from build123d import *

# Parameters (mm, degrees)
X_WING_DEPTH       = 12.7
SKETCH4_3_R        = 1.5
SKETCH4_3_R_2      = 3.175
HOLES_DEPTH        = 9.525
CHIP_DEPTH         = 6.35
EXTRUDE_9V_DEPTH   = 15.24
SKETCH6_3_R        = 1.27
AIR_HOLES_DEPTH    = 9.525
SKETCH7_W          = 7.542953633
SKETCH7_H          = 7.880697826
SKETCH7_H_2        = 6.417139658
SKETCH7_W_2        = 5.741651273
SKETCH7_H_3        = 8.218442018
AIR_SLOTS_DEPTH    = 1.27
CUT_EXTRUDE1_START = 4.572
SKETCH4_5_R        = 1.5
CUT_EXTRUDE1_DEPTH = 0.508


with BuildPart() as part:
    # Sketch2 → Body (revolve)
    with BuildSketch(Plane(origin=(0, 0, 0), x_dir=(0, 0, -1), z_dir=(1, 0, 0))):
        Polygon((4.4704, 13.9065), (0, 12.5857), (0, 0), (-5.08, 0), (-5.08, 49.53), (64.831152593, 49.53), (64.831152593, 39.37), (59.751152593, 39.37), (59.751152593, 44.45), (0, 44.45), (0, 16.4465), (4.4704, 16.4465), align=None)
    revolve(axis=Axis((0, 0, 0), (0, 0, 1)))

    # Sketch4 → X-Wing (cut)
    with BuildSketch(Plane.XY):
        with BuildLine():
            Line((-4.1656, -12.04250002), (-4.1656, -10.483480973))
            ThreePointArc((-4.1656, -10.483480973), (-6.016064494, -6.016064494), (-10.483480973, -4.1656))
            Line((-10.483480973, -4.1656), (-16.265, -4.1656))
            ThreePointArc((-16.265, -4.1656), (-20.4306, 0), (-16.265, 4.1656))
            Line((-16.265, 4.1656), (-12.04250002, 4.1656))
            Line((-12.04250002, 4.1656), (-10.483480973, 4.1656))
            ThreePointArc((-10.483480973, 4.1656), (-6.016064494, 6.016064494), (-4.1656, 10.483480973))
            Line((-4.1656, 10.483480973), (-4.1656, 12.04250002))
            Line((-4.1656, 12.04250002), (-4.1656, 16.265))
            ThreePointArc((-4.1656, 16.265), (0, 20.4306), (4.1656, 16.265))
            Line((4.1656, 16.265), (4.1656, 12.04250002))
            Line((4.1656, 12.04250002), (4.1656, 10.483480973))
            ThreePointArc((4.1656, 10.483480973), (6.016064494, 6.016064494), (10.483480973, 4.1656))
            Line((10.483480973, 4.1656), (12.04250002, 4.1656))
            Line((12.04250002, 4.1656), (16.265, 4.1656))
            ThreePointArc((16.265, 4.1656), (20.4306, 0), (16.265, -4.1656))
            Line((16.265, -4.1656), (12.04250002, -4.1656))
            Line((12.04250002, -4.1656), (10.483480973, -4.1656))
            ThreePointArc((10.483480973, -4.1656), (6.016064494, -6.016064494), (4.1656, -10.483480973))
            Line((4.1656, -10.483480973), (4.1656, -12.04250002))
            Line((4.1656, -12.04250002), (4.1656, -16.265))
            ThreePointArc((4.1656, -16.265), (0, -20.4306), (-4.1656, -16.265))
            Line((-4.1656, -16.265), (-4.1656, -12.04250002))
        make_face()
    extrude(amount=-X_WING_DEPTH, mode=Mode.SUBTRACT)

    # Sketch4<3> → Holes (cut)
    with BuildSketch(Plane.XY):
        with Locations(Location((0, -16.265, 0), (0, 0, 180))):
            Circle(SKETCH4_3_R)
        with Locations(Location((-16.265, 0, 0), (0, 0, 180))):
            Circle(SKETCH4_3_R)
        with Locations(Location((16.265, 0, 0), (0, 0, 180))):
            Circle(SKETCH4_3_R)
        with Locations(Location((0, 16.265, 0), (0, 0, 180))):
            Circle(SKETCH4_3_R)
        with BuildLine():
            ThreePointArc((-7.633217703, 13.021371376), (-7.633217703, 17.511499436), (-12.123345763, 17.511499436))
            Line((-12.123345763, 17.511499436), (-17.511499436, 12.123345763))
            ThreePointArc((-17.511499436, 12.123345763), (-17.511499436, 7.633217703), (-13.021371376, 7.633217703))
            Line((-13.021371376, 7.633217703), (-7.633217703, 13.021371376))
        make_face()
        with Locations((-8.261128525, 8.261128525)):
            Circle(SKETCH4_3_R_2)
        with Locations(Location((8.261128525, 8.261128525, 0), (0, 0, 125.826899667))):
            Circle(SKETCH4_3_R_2)
        with Locations(Location((8.261128525, -8.261128525, 0), (0, 0, 234.173100333))):
            Circle(SKETCH4_3_R_2)
        with Locations(Location((-8.261128525, -8.261128525, 0), (0, 0, 144.173100333))):
            Circle(SKETCH4_3_R_2)
    extrude(amount=HOLES_DEPTH, mode=Mode.SUBTRACT)

    # Sketch6 → Chip (add)
    with BuildSketch(Plane.XY.offset(5.08)):
        Polygon((11.350015507, 22.225), (-11.715690517, 22.225), (-12.954, 22.225), (-12.954, 16.6808452), (-12.7, 16.9348452), (-12.7, 20.32), (12.7, 20.32), (12.7, -20.32), (-12.7, -20.32), (-12.7, 7.954589078), (-12.954, 7.700589078), (-12.954, -22.225), (12.954, -22.225), (12.954, 22.225), align=None)
    extrude(amount=CHIP_DEPTH)

    # Sketch6<4> → Extrude 9V (add)
    with BuildSketch(Plane.XY.offset(5.08)):
        Polygon((-14.859, 14.7758452), (-12.954, 16.6808452), (-12.954, 22.225), (-11.715690517, 22.225), (-11.715690517, 23.479848526), (-14.859, 23.479848526), align=None)
        with BuildLine():
            ThreePointArc((-13.021371376, 7.633217703), (-13.865328691, 7.029154679), (-14.859, 6.729532555))
            Line((-14.859, 6.729532555), (-14.859, 0.522650935))
            ThreePointArc((-14.859, 0.522650935), (-14.765, 0), (-14.859, -0.522650935))
            Line((-14.859, -0.522650935), (-14.859, -24.638))
            Line((-14.859, -24.638), (14.859, -24.638))
            Line((14.859, -24.638), (14.859, -0.522650935))
            ThreePointArc((14.859, -0.522650935), (14.765, 0), (14.859, 0.522650935))
            Line((14.859, 0.522650935), (14.859, 29.972))
            Line((14.859, 29.972), (-14.859, 29.972))
            Line((-14.859, 29.972), (-14.859, 28.067))
            Line((-14.859, 28.067), (12.954, 28.067))
            Line((12.954, 28.067), (12.954, 23.734213344))
            Line((12.954, 23.734213344), (11.350015507, 23.734213344))
            Line((11.350015507, 23.734213344), (11.350015507, 22.225))
            Line((11.350015507, 22.225), (12.954, 22.225))
            Line((12.954, 22.225), (12.954, -22.733))
            Line((12.954, -22.733), (-12.954, -22.733))
            Line((-12.954, -22.733), (-12.954, 7.700589078))
            Line((-12.954, 7.700589078), (-13.021371376, 7.633217703))
        make_face()
    extrude(amount=EXTRUDE_9V_DEPTH)

    # Sketch6<3> → Air holes (cut)
    with BuildSketch(Plane.XY.offset(5.08)):
        with Locations((-23.749, -23.368)):
            Circle(SKETCH6_3_R)
        with Locations((23.114, -15.748)):
            Circle(SKETCH6_3_R)
        with Locations((-9.906, 36.322)):
            Circle(SKETCH6_3_R)
        with Locations((18.034, 36.322)):
            Circle(SKETCH6_3_R)
    extrude(amount=-AIR_HOLES_DEPTH, mode=Mode.SUBTRACT)

    # Sketch7 → Air Slots (cut)
    with BuildSketch(Plane.XY.offset(5.08)):
        with Locations((15.537525525, 8.731732869)):
            Rectangle(SKETCH7_W, SKETCH7_H)
        with Locations((15.537525525, -8.324348854)):
            Rectangle(SKETCH7_W, SKETCH7_H_2)
        with Locations((-14.859451804, -9.225000034)):
            Rectangle(SKETCH7_W_2, SKETCH7_H_3)
    extrude(amount=AIR_SLOTS_DEPTH, mode=Mode.SUBTRACT)

    # SurfaceCut1
    split(bisect_by=Plane.XY.offset(5.08), keep=Keep.BOTTOM)

    # Sketch4<5> → Cut-Extrude1 (cut)
    with BuildSketch(Plane.XY.offset(CUT_EXTRUDE1_START)):
        with BuildLine():
            ThreePointArc((5.098211557, -7.98439534), (6.016064494, -6.016064494), (7.98439534, -5.098211557))
            ThreePointArc((7.98439534, -5.098211557), (9.203861468, -4.686142824), (10.483480973, -4.5466))
            Line((10.483480973, -4.5466), (16.265, -4.5466))
            ThreePointArc((16.265, -4.5466), (20.8116, 0), (16.265, 4.5466))
            Line((16.265, 4.5466), (10.483480973, 4.5466))
            ThreePointArc((10.483480973, 4.5466), (9.203861468, 4.686142824), (7.98439534, 5.098211557))
            ThreePointArc((7.98439534, 5.098211557), (6.016064494, 6.016064494), (5.098211557, 7.98439534))
            ThreePointArc((5.098211557, 7.98439534), (4.686142824, 9.203861468), (4.5466, 10.483480973))
            Line((4.5466, 10.483480973), (4.5466, 16.265))
            ThreePointArc((4.5466, 16.265), (0, 20.8116), (-4.5466, 16.265))
            Line((-4.5466, 16.265), (-4.5466, 10.483480973))
            ThreePointArc((-4.5466, 10.483480973), (-4.686142824, 9.203861468), (-5.098211557, 7.98439534))
            ThreePointArc((-5.098211557, 7.98439534), (-6.016064494, 6.016064494), (-7.98439534, 5.098211557))
            ThreePointArc((-7.98439534, 5.098211557), (-9.203861468, 4.686142824), (-10.483480973, 4.5466))
            Line((-10.483480973, 4.5466), (-16.265, 4.5466))
            ThreePointArc((-16.265, 4.5466), (-20.8116, 0), (-16.265, -4.5466))
            Line((-16.265, -4.5466), (-10.483480973, -4.5466))
            ThreePointArc((-10.483480973, -4.5466), (-9.203861468, -4.686142824), (-7.98439534, -5.098211557))
            ThreePointArc((-7.98439534, -5.098211557), (-6.016064494, -6.016064494), (-5.098211557, -7.98439534))
            ThreePointArc((-5.098211557, -7.98439534), (-4.686142824, -9.203861468), (-4.5466, -10.483480973))
            Line((-4.5466, -10.483480973), (-4.5466, -16.265))
            ThreePointArc((-4.5466, -16.265), (0, -20.8116), (4.5466, -16.265))
            Line((4.5466, -16.265), (4.5466, -10.483480973))
            ThreePointArc((4.5466, -10.483480973), (4.686142824, -9.203861468), (5.098211557, -7.98439534))
        make_face()
        with Locations(Location((0, -16.265, 0), (0, 0, 180))):
            Circle(SKETCH4_5_R, mode=Mode.SUBTRACT)
        with Locations(Location((16.265, 0, 0), (0, 0, 180))):
            Circle(SKETCH4_5_R, mode=Mode.SUBTRACT)
        with Locations(Location((-16.265, 0, 0), (0, 0, 180))):
            Circle(SKETCH4_5_R, mode=Mode.SUBTRACT)
        with Locations(Location((0, 16.265, 0), (0, 0, 180))):
            Circle(SKETCH4_5_R, mode=Mode.SUBTRACT)
    extrude(amount=CUT_EXTRUDE1_DEPTH, mode=Mode.SUBTRACT)


solid = part.part
Design review of the part built by this model. Coordinates are the model's own, in mm. A direction names the side the tool comes from. Round coordinates to 2 decimals unless told otherwise and drop trailing zeros. Write each loop counter-clockwise with the first axis right and the second up, starting at its lowest first coordinate (ties: lowest second). Pieces come first, ordered by that corner, then holes. Notation, with made-up numbers: (-13.5, 60) -> (25.5, 60) arc R21 cw to (25.5, 82) -> close; hole circle Ø8 at (36, 13.5). An arc over 180 degrees is marked (long way). One line per item, written item: value. Start each with the question number.
Q1. Tool access review of faces 3 (the face through (11.72, 11.54, -2.27)), 4 (the face through (0.1, 20.81, 4.82)), 5 (the face through (29, 27, -59.751)), 6 (the face through (14.834, -0.451, 2.254)): name each direction out of +Z, -Z, +X, -X, +Y, -Y from which nothing blocks a thin tool from reaching the whole face with its end or side.
Q2. Add section A-A (x = 0). Give the boundary of the cut face in (y, z) (3 decimals).
Q3. To check wall thickness, follow probe 1 along Y at (x, z) = (0, 2.5) (3 decimals); probe 2 along Z at (x, y) = (-42.5, -9); probe 3 along Z at (x, y) = (-26.5, 12). State the ranges of each line that lie inside material, in increasing order.
Q4. Add section C-C (y = -38). Give the boundary of the cut face in (x, z), then the cut area to 3 significant figures.
Q5. Insertion check: P1, Ø3.5, axis at x = -16.265, y = 0, coming from the +Z side; P2, Ø7, axis at x = -10, y = 12.5, coming from the +Z side; P3, Ø0.6, axis at x = -13, z = 5, coming from the +Y side; P4, Ø5, axis at x = 8.26, y = -8.26, coming from the -Z side. Each pin has a flat end and moves straight along its axis. Give the tip position at first contact, or say it passes through.
Q6. The part is to be moulded in two halves that separate along X. For faces 1 (the face through (-10, -11, -4.47)), 2 (the face through (10, 10, -4.47)), say which applies: pulls with the +X half, pulls with the -X half, needs draft (parallel to the pull), parting line crosses it, or undercut.
Q7. Add section D-D (x = 28). Give the boundary of the cut face in (y, z).
Response:
1. face 3: -Z
1. face 4: +Z
1. face 5: none
1. face 6: +Z, -Z
2. outline: (-49.53, -64.831) -> (-39.37, -64.831) -> (-39.37, -59.751) -> (-44.45, -59.751) -> (-44.45, 0) -> (-17.765, 0) -> (-17.765, 4.572) -> (-20.812, 4.572) -> (-20.812, 5.08) -> (-49.53, 5.08) -> close; (-14.765, 0) -> (14.765, 0) -> (14.765, 4.572) -> (-14.765, 4.572) -> close; (17.765, 0) -> (44.45, 0) -> (44.45, -59.751) -> (39.37, -59.751) -> (39.37, -64.831) -> (49.53, -64.831) -> (49.53, 5.08) -> (20.812, 5.08) -> (20.812, 4.572) -> (17.765, 4.572) -> close
3. probe 1: y = -49.53 to -17.765, -14.765 to 14.765, 17.765 to 49.53
3. probe 2: z = -64.83 to -59.75, 0 to 5.08
3. probe 3: z = 0 to 5.08
4. outline: (-31.77, -64.83) -> (-10.3, -64.83) -> (-10.3, -59.75) -> (-23.06, -59.75) -> (-23.06, 0) -> (23.06, 0) -> (23.06, -59.75) -> (10.3, -59.75) -> (10.3, -64.83) -> (31.77, -64.83) -> (31.77, 5.08) -> (-31.77, 5.08) -> close
4. area: 1,580 mm^2
5. P1: stops at z = 4.57
5. P2: stops at z = 5.08
5. P3: stops at y = 47.87
5. P4: stops at z = -4.47
6. face 1: undercut
6. face 2: undercut
7. outline: (-40.86, -64.83) -> (-27.68, -64.83) -> (-27.68, -59.75) -> (-34.52, -59.75) -> (-34.52, 0) -> (34.52, 0) -> (34.52, -59.75) -> (27.68, -59.75) -> (27.68, -64.83) -> (40.86, -64.83) -> (40.86, 5.08) -> (-40.86, 5.08) -> close
